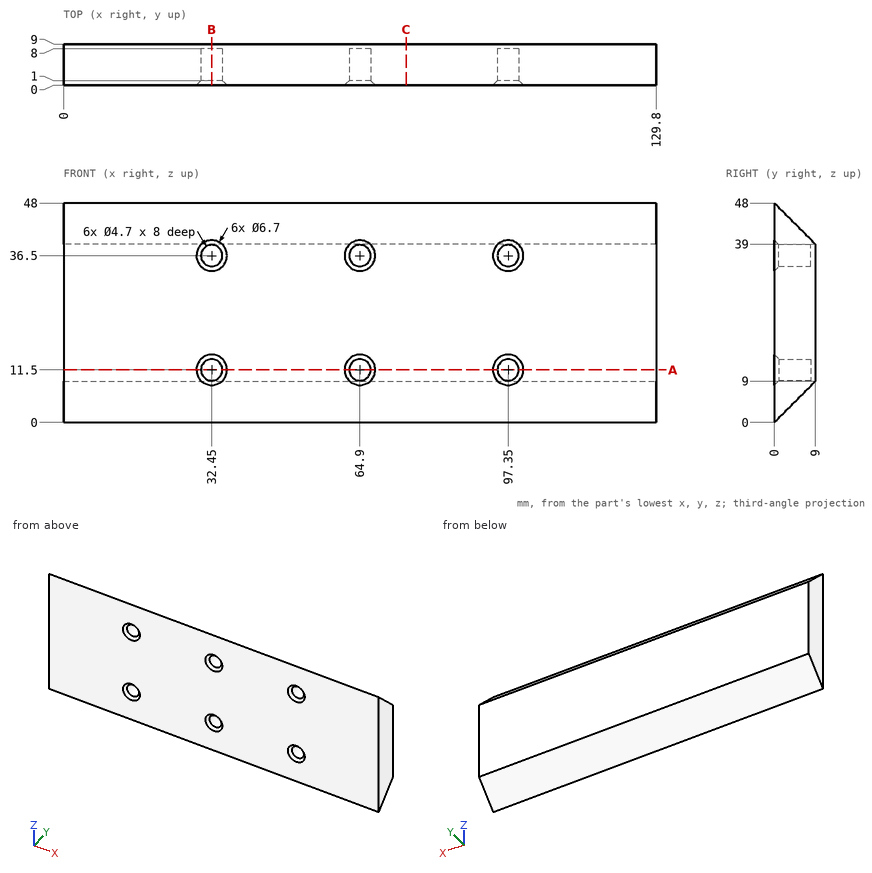
Could you check a few things on this drawing? It's one solid part, dimensions in mm from its lowest x, y, z. Coordinates: 2 decimals unless noted, no trailing zeros. Write each loop counter-clockwise with the first axis right and the second up, starting at its lowest first coordinate (ties: lowest second). Pieces come first, ordered by that corner, then holes. Notation, with made-up numbers: (-32, 6) - (-15, 6) arc R20 cw to (-15, 38) - close; hole circle Ø5 at (2.5, 84.25). An arc over 180 degrees is marked (long way). Put each result on its own line as item: value. Start each with the question number.
Q1. I want a section at A-A on z = 11.5. Write out the boundary of the cut face in (x, y), plus the area to 3 significant figures.
Q2. I want a section at B-B on x = 32.45. Write out the boundary of the cut face in (y, z), plus the area to 3 significant figures.
Q3. I want a section at C-C on x = 75. Write out the boundary of the cut face in (y, z), plus the area to 3 significant figures.
Q4. I'm going to push flat-ended pins straight in: P1, Ø1.4, axis at x = 65.5, z = 36.5, coming from the -Y side; P2, Ø4, axis at x = 16.5, z = 36.5, coming from the -Y side; P3, Ø5.5, axis at x = 64.9, z = 11.5, coming from the -Y side; P4, Ø5, axis at x = 23.5, y = 7, coming from the +Z side. Where does each tip first touch, or does it pass through?
Q5. Please list where these lines run through material, in increasing order: L1, parallel to X at y = 5.5, z = 36.5; L2, parallel to X at y = 4.5, z = 10; L3, parallel to Z at x = 64, y = 6.
Checks:
1. outline: (0, 0) - (29.1, 0) - (30.1, 1) - (30.1, 8) - (34.8, 8) - (34.8, 1) - (35.8, 0) - (61.55, 0) - (62.55, 1) - (62.55, 8) - (67.25, 8) - (67.25, 1) - (68.25, 0) - (94, 0) - (95, 1) - (95, 8) - (99.7, 8) - (99.7, 1) - (100.7, 0) - (129.8, 0) - (129.8, 9) - (0, 9) - close
1. area: 1,050 mm²
2. outline: (0, 0) - (9, 9) - (9, 39) - (0, 48) - (0, 39.85) - (1, 38.85) - (8, 38.85) - (8, 34.15) - (1, 34.15) - (0, 33.15) - (0, 14.85) - (1, 13.85) - (8, 13.85) - (8, 9.15) - (1, 9.15) - (0, 8.15) - close
2. area: 274 mm²
3. outline: (0, 0) - (9, 9) - (9, 39) - (0, 48) - close
3. area: 351 mm²
4. P1: y = 8
4. P2: y = 0
4. P3: y = 0.6
4. P4: z = 43.5
5. L1: 0 to 30.1, 34.8 to 62.55, 67.25 to 95, 99.7 to 129.8
5. L2: 0 to 30.64, 34.26 to 63.09, 66.71 to 95.54, 99.16 to 129.8
5. L3: 6 to 9.33, 13.67 to 34.33, 38.67 to 42
